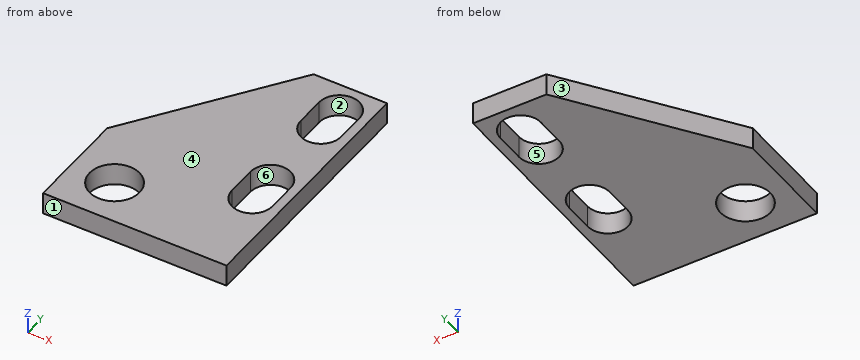
```python
from build123d import *

# Parameters (mm, degrees)
F0_W     = 25
F0_H     = 35
F1_DEPTH = 3
F3_DEPTH = 25
F4_D     = 6.8
F4_DEPTH = 16.35
F4_TIP   = 2.0429261047
F6_DEPTH = 25


with BuildPart() as f1:
    # F0 (on Top) → F1 (new body)
    with BuildSketch(Plane.XY):
        with Locations((12.5, -17.5)):
            Rectangle(F0_W, F0_H)
    extrude(amount=F1_DEPTH)

    # F2 (on face) → F3 (cut)
    with BuildSketch(Plane.XY.offset(3)):
        with BuildLine():
            Line((18.25, -4), (23.75, -4))
            ThreePointArc((23.75, -4), (21, -1.25), (18.25, -4))
        make_face()
        with BuildLine():
            Line((23.75, -8), (23.75, -4))
            ThreePointArc((23.75, -4), (23.5251743677, -5.089033706), (22.8874586088, -6))
            ThreePointArc((22.8874586088, -6), (23.5251743677, -6.910966294), (23.75, -8))
        make_face()
        with BuildLine():
            ThreePointArc((22.8874586088, -6), (23.5251743677, -5.089033706), (23.75, -4))
            Line((23.75, -4), (18.25, -4))
            ThreePointArc((18.25, -4), (18.4748256323, -5.089033706), (19.1125413912, -6))
            ThreePointArc((19.1125413912, -6), (21, -5.25), (22.8874586088, -6))
        make_face()
        with BuildLine():
            ThreePointArc((19.1125413912, -6), (18.4748256323, -5.089033706), (18.25, -4))
            Line((18.25, -4), (18.25, -8))
            ThreePointArc((18.25, -8), (18.4748256323, -6.910966294), (19.1125413912, -6))
        make_face()
        with BuildLine():
            ThreePointArc((23.75, -8), (23.5251743677, -6.910966294), (22.8874586088, -6))
            ThreePointArc((22.8874586088, -6), (21, -6.75), (19.1125413912, -6))
            ThreePointArc((19.1125413912, -6), (18.4748256323, -6.910966294), (18.25, -8))
            ThreePointArc((18.25, -8), (21, -10.75), (23.75, -8))
        make_face()
        with BuildLine():
            ThreePointArc((22.8874586088, -21), (23.5251743677, -20.089033706), (23.75, -19))
            ThreePointArc((23.75, -19), (21, -16.25), (18.25, -19))
            ThreePointArc((18.25, -19), (18.4748256323, -20.089033706), (19.1125413912, -21))
            ThreePointArc((19.1125413912, -21), (21, -20.25), (22.8874586088, -21))
        make_face()
        with BuildLine():
            Line((23.75, -23), (23.75, -19))
            ThreePointArc((23.75, -19), (23.5251743677, -20.089033706), (22.8874586088, -21))
            ThreePointArc((22.8874586088, -21), (23.5251743677, -21.910966294), (23.75, -23))
        make_face()
        with BuildLine():
            ThreePointArc((19.1125413912, -21), (18.4748256323, -20.089033706), (18.25, -19))
            Line((18.25, -19), (18.25, -23))
            ThreePointArc((18.25, -23), (18.4748256323, -21.910966294), (19.1125413912, -21))
        make_face()
        with BuildLine():
            ThreePointArc((23.75, -23), (23.5251743677, -21.910966294), (22.8874586088, -21))
            ThreePointArc((22.8874586088, -21), (21, -21.75), (19.1125413912, -21))
            ThreePointArc((19.1125413912, -21), (18.4748256323, -21.910966294), (18.25, -23))
            ThreePointArc((18.25, -23), (21, -25.75), (23.75, -23))
        make_face()
        with BuildLine():
            ThreePointArc((19.1125413912, -21), (21, -21.75), (22.8874586088, -21))
            ThreePointArc((22.8874586088, -21), (21, -20.25), (19.1125413912, -21))
        make_face()
        with BuildLine():
            ThreePointArc((19.1125413912, -6), (21, -6.75), (22.8874586088, -6))
            ThreePointArc((22.8874586088, -6), (21, -5.25), (19.1125413912, -6))
        make_face()
    extrude(amount=-F3_DEPTH, mode=Mode.SUBTRACT)

    # F4
    with Locations(Plane.XY.offset(3)):
        with Locations((6, -29)):
            Hole(F4_D / 2, depth=F4_DEPTH)
            with Locations((0, 0, -(F4_DEPTH + F4_TIP / 2))):  # 118° drill point
                Cone(0, F4_D / 2, F4_TIP, mode=Mode.SUBTRACT)

    # F5 (on face) → F6 (cut)
    with BuildSketch(Plane.XY.offset(3)):
        Polygon((0, -21), (15, 0), (0, 0), align=None)
    extrude(amount=-F6_DEPTH, mode=Mode.SUBTRACT)


solid = f1.part
```
Build history of the part. All positions in model axes, mm. Face numbers are marked on the shaded views. A direction names the side the tool comes from. Round coordinates to 2 decimals unless told otherwise and drop trailing zeros. Loops run counter-clockwise (first coordinate to the right, second up) from the corner with the lowest first, then second, coordinate; pieces in that order, holes last.
Item 1: Saw through at A-A (x = 21). List the corners of the cut face in (y, z), then the cut area to 3 significant figures.
Item 2: Which spindle directions (+Z, -Z, +X, -X, +Y, -Y) get a long thin tool onto all of the face, cutting with end or side? Do the marked faces 1 and 2. Say none if no direction does.
Item 3: Saw through at C-C (z = 2.2). List the corners of the cut face in (x, y), then the cut area to 3 significant figures.
Item 4: Saw through at D-D (x = 6). List the corners of the cut face in (y, z), then the cut area to 3 significant figures.
Item 5: Saw through at B-B (y = -29). List the corners of the cut face in (x, z), then the cut area to 3 significant figures.
Item 6: Pin check, flat tip, straight feed: P1, Ø6, axis at x = 6, y = -29, coming from the +Z side. Stop position of the tip, or through.
Item 7: Two-plate mould, pull along X, no slides. Class the marked faces 3, 4, 5 and 6: released by +X, released by -X, zero draft, split by the parting line, or undercut.
Item 8: Drill centre lines: line 1 along Y through (x, z) = (21.5, 0.9); line 2 along X through (y, z) = (-21, 1.15); line 3 along Y through (x, z) = (4, 2.35). Where is each one in solid material? Low to high.
Worked answers:
1. outline: (-35, 0) - (-25.75, 0) - (-25.75, 3) - (-35, 3) - close; (-16.25, 0) - (-10.75, 0) - (-10.75, 3) - (-16.25, 3) - close; (-1.25, 0) - (0, 0) - (0, 3) - (-1.25, 3) - close
1. area: 48.0 mm2
2. face 1: +Z, -Z, +X, -X, -Y
2. face 2: +Z, -Z
3. outline: (0, -35) - (25, -35) - (25, 0) - (15, 0) - (0, -21) - close; hole circle Ø6.8 at (6, -29); hole (18.25, -23) arc R2.75 ccw to (23.75, -23) - (23.75, -19) arc R2.75 ccw to (18.25, -19) - close; hole (18.25, -8) arc R2.75 ccw to (23.75, -8) - (23.75, -4) arc R2.75 ccw to (18.25, -4) - close
3. area: 590 mm2
4. outline: (-35, 0) - (-32.4, 0) - (-32.4, 3) - (-35, 3) - close; (-25.6, 0) - (-12.6, 0) - (-12.6, 3) - (-25.6, 3) - close
4. area: 46.8 mm2
5. outline: (0, 0) - (2.6, 0) - (2.6, 3) - (0, 3) - close; (9.4, 0) - (25, 0) - (25, 3) - (9.4, 3) - close
5. area: 54.6 mm2
6. P1: passes through
7. face 3: released by -X
7. face 4: zero draft
7. face 5: undercut
7. face 6: undercut
8. line 1: y = -35 to -25.7, -16.3 to -10.7, -1.3 to 0
8. line 2: x = 0 to 18.25, 23.75 to 25
8. line 3: y = -35 to -31.75, -26.25 to -15.4
